Autodesk Inventor part; units mm, degrees
ref_plane "YZ Plane" through (0, 0, 0) normal (1, 0, 0) x (0, 1, 0)
ref_plane "XZ Plane" through (0, 0, 0) normal (0, 1, 0) x (-1, 0, 0)
ref_plane "XY Plane" through (0, 0, 0) normal (0, 0, 1) x (1, 0, 0)
sketch "Sketch1" plane through (0, 0, 0) normal (0, 1, 0) x (-1, 0, 0)
  circle A0 centre (0, 0) radius 4
  dimension "d0" = 8
extrude "Extrusion1" add sketch "Sketch1" along normal blind 64
sketch "Sketch2" plane through (0, 64, 0) normal (0, 1, 0) x (1, 0, 0)
  point P0 (0, 0)
  point P1 (0, 0)
sketch "Sketch3" plane through (0, 0, 0) normal (0, -1, 0) x (1, 0, 0)
  point P0 (0, 0)
  point P1 (0, 0)
hole "Hole1" at (0, 64, 0) direction (0, -1, 0) diameter 2.459 depth 10.8 tip angle 118
hole "Hole2" at (0, 0, 0) direction (0, 1, 0) diameter 2.459 depth 10.8 tip angle 118
properties part number "rod"
Geometry: final body of the model. Coordinates: model frame, mm. A direction names the side the tool comes from. Give positions to 0.01 mm unless a question says otherwise; leave off trailing zeros. Order: outer loops, then holes, each group sorted by start corner. A loop starts at its lowest first (then second) coordinate and runs counter-clockwise, first axis right, second up. Notation, with made-up numbers: M 15.5,-25 L 20.5,-25 A19 ccw 20.5,2 Z; hole C 34.25,3 d11. An arc over 180 degrees is marked long. Answer as CSV lines item,"result". Start each with the question number.
1) Mould query, pull axis Z, two halves, no side actions, for faces 4 (the cylindrical face through (0.867, 31.552, 3.905)), 5 (the flat face through (1, 64, -1)), 6 (the conical face through (-0.08, 52.59, 0.2)). Classes: +Z half, -Z half, draft (parallel to the pull), parting line (faces both ways), or undercut.
2) Cut plane B-B (z = 2). Output: boundary loops of the cut face in (x, y), then the cut area to 3 significant figures.
3) Line query: line 1 (Z direction, x = 0, y = 7.5); line 2 (Z direction, x = 1, y = 56); line 3 (X direction, y = 7, z = 0.25). Output: solid intervals per line, ascending. Write a range as from..to.
4) Cut plane A-A (y = 40). Output: boundary loops of the cut face in (x, z).
5) Cut plane C-C (x = -2). Output: boundary loops of the cut face in (y, z).
6) First-contact query: P1, Ø1.5, axis at x = 1.5, y = 49.5, coming from the -Z side. Flat tip, straight axial feed; report the tip coordinate or a pass-through.
7) Set-up query: faces 1 (the cylindrical face through (0.748, 5.476, 0.976)), 2 (the cylindrical face through (0.748, 58.524, -0.976)), 3 (the flat face through (1, 0, -1)). Return all of +Z, -Z, +X, -X, +Y, -Y with unobstructed straight access to the full face (end or side cutting, diameter ignored); none if empty.
Findings below:
1,face 4,"parting line"
1,face 5,"draft"
1,face 6,"undercut"
2,outline,"M -3.46,0 L 3.46,0 L 3.46,64 L -3.46,64 Z"
2,area,"443 mm²"
3,line 1,"z = -4..-1.23, 1.23..4"
3,line 2,"z = -3.87..-0.72, 0.72..3.87"
3,line 3,"x = -3.99..-1.2, 1.2..3.99"
4,outline,"C 0,0 d8"
5,outline,"M 0,-3.46 L 64,-3.46 L 64,3.46 L 0,3.46 Z"
6,P1,"stops at z = -3.93"
7,face 1,"-Y"
7,face 2,"+Y"
7,face 3,"+Z, -Z, +X, -X, -Y"
